Check sheet for the modelled part. Datum: model origin and axes. Units: mm. Face numbers are marked on the shaded views. A direction names the side the tool comes from. Round coordinates to 2 decimals unless told otherwise and drop trailing zeros. Loops run counter-clockwise (first coordinate to the right, second up) from the corner with the lowest first, then second, coordinate; pieces in that order, holes last. Notation, with made-up numbers: (45, -26.75) - (82, -26.75) arc R24 cw to (82, 8.25) - close; hole circle Ø7 at (70.5, 22). An arc over 180 degrees is marked (long way). Put each result on its own line as item: value. Start each with the question number.
Item 1: Section check B-B, the plane y = 4. Record the cut outline in (x, z), and give its area (3 significant figures).
Item 2: Gauge pin test, flat ends, axial feed: pin 1 Ø5.5 at (x, y) = (-29, 8) entering from -Z; pin 2 Ø1.5 at (x, y) = (-28, 6) entering from +Z; pin 3 Ø5 at (y, z) = (9.5, 16) entering from -X; pin 4 Ø1.5 at (x, z) = (-19.5, 20) entering from -Y. Record the tip position at first contact, or that the pin passes through.
Item 3: Tool access check on the marked faces 1, 2, 3 and 4. Record the directions out of +Z, -Z, +X, -X, +Y, -Y that give a thin tool (end or side, any length) a straight path to the whole face; none if there is none.
Item 4: Material ranges on line 1 along Z through (x, y) = (0.5, 13.5); line 2 along X through (y, z) = (4.25, 3); line 3 along X through (y, z) = (10, -8.5), recorded low to high.
Item 5: Section check C-C, the plane y = 7.5. Record the cut outline in (x, z) (3 decimals).
from build123d import *

# Parameters (mm, degrees)
BOSS_EXTRUDE1_DEPTH = 15
REVOLVE2_ANGLE      = 347.2
SKETCH9_R           = 1.25
CUT_EXTRUDE1_DEPTH  = 20
SKETCH10_R          = 2.475
CUT_EXTRUDE3_DEPTH  = 4
SKETCH12_R          = 1
CUT_EXTRUDE4_DEPTH  = 5
SKETCH13_R          = 2.5
CUT_EXTRUDE6_DEPTH  = 24
CHAMFER1_SIZE       = 0.2
FILLET1_R           = 1
CHAMFER2_SIZE       = 0.5
CHAMFER3_SIZE       = 2


with BuildPart() as part:
    # Sketch3 → Boss-Extrude1 (new body)
    with BuildSketch(Plane(origin=(0, 0, 0), x_dir=(1, 0, 0), z_dir=(0, 1, 0))):
        with BuildLine():
            Line((22.360679775, 2.5), (37.360679775, 2.5))
            Line((37.360679775, 2.5), (37.360679775, 7.5))
            Line((37.360679775, 7.5), (28.530685235, 7.5))
            ThreePointArc((28.530685235, 7.5), (0.890802954, 29.486547273), (-28.025910222, 9.208602294))
            Line((-28.025910222, 9.208602294), (-30.781929629, 9.208602294))
            Line((-30.781929629, 9.208602294), (-30.781929629, -9.208602294))
            Line((-30.781929629, -9.208602294), (-28.025910222, -9.208602294))
            ThreePointArc((-28.025910222, -9.208602294), (0.890802954, -29.486547273), (28.530685235, -7.5))
            Line((28.530685235, -7.5), (37.360679775, -7.5))
            Line((37.360679775, -7.5), (37.360679775, -2.5))
            Line((37.360679775, -2.5), (22.360679775, -2.5))
            ThreePointArc((22.360679775, -2.5), (-22.5, 0), (22.360679775, 2.5))
        make_face()
    extrude(amount=BOSS_EXTRUDE1_DEPTH)

    # Sketch8 → Revolve2 (revolve)
    with BuildSketch(Plane(origin=(0, 0, 0), x_dir=(-0.9938079899999066, 0, 0.11111111111111108), z_dir=(-0.11111111111111106, 0, -0.9938079899999065))):
        Polygon((-22.5, 9), (-21.33, 9), (-21.33, 10.45), (-22.04, 10.45), (-22.04, 15), (-22.5, 15), align=None)
    revolve(axis=Axis((0, 0, 0), (0, 1, 0)), revolution_arc=REVOLVE2_ANGLE)

    # Sketch9 → Cut-Extrude1 (cut)
    with BuildSketch(Plane.XY.offset(7.5)):
        with Locations((32.945682505, 11)):
            Circle(SKETCH9_R)
        with Locations((32.945682505, 4)):
            Circle(SKETCH9_R)
    extrude(amount=-CUT_EXTRUDE1_DEPTH, mode=Mode.SUBTRACT)

    # Sketch10 → Cut-Extrude3 (cut)
    with BuildSketch(Plane.ZY.offset(30.781929629)):
        with Locations((0, 7.5)):
            Circle(SKETCH10_R)
    extrude(amount=-CUT_EXTRUDE3_DEPTH, mode=Mode.SUBTRACT)

    # Sketch12 → Cut-Extrude4 (cut)
    with BuildSketch(Plane.ZY.offset(26.781929629)):
        with Locations((0, 7.5)):
            Circle(SKETCH12_R)
    extrude(amount=-CUT_EXTRUDE4_DEPTH, mode=Mode.SUBTRACT)

    # Sketch13 → Cut-Extrude6 (cut)
    with BuildSketch(Plane(origin=(0, 0, 0), x_dir=(0, 0, -1), z_dir=(1, 0, 0))):
        with Locations((0, 7.5)):
            Circle(SKETCH13_R)
    extrude(amount=-CUT_EXTRUDE6_DEPTH, mode=Mode.SUBTRACT)

    # Chamfer1
    chamfer1_edges = [part.edges().sort_by_distance(p)[0] for p in [
        (-0.259360391, 9, 22.49850511),
        (-22.039998571, 10.45, -0.007935673),
    ]]
    chamfer(chamfer1_edges, length=CHAMFER1_SIZE)

    # Fillet1
    fillet1_edges = [part.edges().sort_by_distance(p)[0] for p in [
        (28.530685235, 7.5, 7.5),
        (28.530685235, 7.5, -7.5),
    ]]
    fillet(fillet1_edges, radius=FILLET1_R)

    # Chamfer2
    # the kernel refuses this chamfer: 0.5 mm, written as the material it takes off along each edge
    with BuildSketch(Plane(origin=(0, 10.45, 0), x_dir=(0.9987152347198149, 0, -0.05067425321151771), z_dir=(0.05067425321151771, 0, 0.9987152347198149))) as chamfer2_piece_1:
        Polygon((21.33, -CHAMFER2_SIZE), (21.33 + CHAMFER2_SIZE, 0), (21.33, 0), align=None)
    revolve(axis=Axis((0, 10.45, 0), (0, 1, 0)), revolution_arc=354.149410651, mode=Mode.SUBTRACT)

    # Chamfer3
    chamfer3_edges = [part.edges().sort_by_distance(p)[0] for p in [
        (0.516715321, 0, -29.495474319),
        (33.326158403, 0, 7.5),
        (28.691090832, 0, -7.700409941),
        (28.691090832, 0, 7.700409941),
        (0.516715321, 0, 29.495474319),
        (33.326158403, 0, -7.5),
    ]]
    chamfer(chamfer3_edges, length=CHAMFER3_SIZE)


solid = part.part
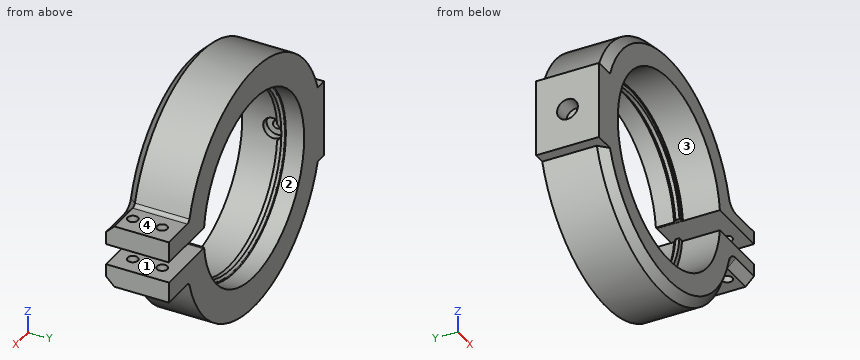
Check result:
1. outline: (-30.78, -9.21) - (-28.03, -9.21) arc R29.5 ccw to (28.33, -8.22) arc R1 cw to (29.29, -7.5) - (31.7, -7.5) - (31.7, -2.5) - (22.36, -2.5) arc R22.5 cw (long way) to (22.36, 2.5) - (31.7, 2.5) - (31.7, 7.5) - (29.29, 7.5) arc R1 cw to (28.33, 8.22) arc R29.5 ccw to (-28.03, 9.21) - (-30.78, 9.21) - close; (34.2, -7.5) - (37.36, -7.5) - (37.36, -2.5) - (34.2, -2.5) - close; (34.2, 2.5) - (37.36, 2.5) - (37.36, 7.5) - (34.2, 7.5) - close
1. area: 1,200 mm²
2. pin 1: z = -13.46
2. pin 2: z = 11.3
2. pin 3: x = -26.23
2. pin 4: y = 0
3. face 1: +X, +Y, -Y
3. face 2: +Y
3. face 3: -Y
3. face 4: +Z, +X, +Y, -Y
4. line 1: -29.5 to -22.03, 22.03 to 29.5
4. line 2: -30.78 to -22.3, 22.3 to 31.72, 34.17 to 37.36
4. line 3: -30.78 to -19.62, 19.62 to 28.25
5. outline: (-30.782, -9.209) - (-28.026, -9.209) arc R29.5 ccw to (28.331, -8.221) arc R1 cw to (29.292, -7.5) - (37.361, -7.5) - (37.361, -2.5) - (22.361, -2.5) arc R22.5 cw to (-22.361, -2.5) - (-24, -2.5) - (-24, -1) - (-26.782, -1) - (-26.782, -2.475) - (-30.782, -2.475) - close; (-30.782, 2.475) - (-26.782, 2.475) - (-26.782, 1) - (-24, 1) - (-24, 2.5) - (-22.361, 2.5) arc R22.5 cw to (22.361, 2.5) - (37.361, 2.5) - (37.361, 7.5) - (29.292, 7.5) arc R1 cw to (28.331, 8.221) arc R29.5 ccw to (-28.026, 9.209) - (-30.782, 9.209) - close
